Read the model definition and answer for the solid it produces. Units are mm, in the model's axes. A direction names the side the tool comes from. Give positions to 0.01 mm unless a question says otherwise; leave off trailing zeros. Write each loop counter-clockwise with the first axis right and the second up, starting at its lowest first coordinate (ties: lowest second). Pieces come first, ordered by that corner, then holes. Notation, with made-up numbers: (32, 39) - (55, 39) arc R7 cw to (55, 43) - close; hole circle Ø7 at (-35.75, 60). An arc over 180 degrees is marked (long way). Answer as a JSON object with one key per item and string values. Group by question number.
```python
from build123d import *

# Parameters (mm, degrees)
EXTRUDE_THIN1_DEPTH      = 640
EXTRUDE_THIN1_DEPTH_BACK = 640
CUT_EXTRUDE1_DEPTH       = 644.506021728
CUT_EXTRUDE1_DEPTH_BACK  = 644.506021728
SKETCH2_R                = 9


with BuildPart() as part:
    # Sketch1 → Extrude-Thin1 (new, two sides: drawn at the far end of the back side and taken through both)
    with BuildSketch(Plane(origin=(0, 0, 0), x_dir=(0, 0, -1), z_dir=(1, 0, 0)).offset(-EXTRUDE_THIN1_DEPTH_BACK)):
        with BuildLine():
            Line((-30, 50), (-30, -50))
            ThreePointArc((-30, -50), (-27.071067812, -57.071067812), (-20, -60))
            Line((-20, -60), (20, -60))
            ThreePointArc((20, -60), (27.071067812, -57.071067812), (30, -50))
            Line((30, -50), (30, 50))
            ThreePointArc((30, 50), (27.071067812, 57.071067812), (20, 60))
            Line((20, 60), (-20, 60))
            ThreePointArc((-20, 60), (-27.071067812, 57.071067812), (-30, 50))
        make_face()
        with BuildLine():
            Line((-27, 50), (-27, -50))
            ThreePointArc((-27, -50), (-24.949747468, -54.949747468), (-20, -57))
            Line((-20, -57), (20, -57))
            ThreePointArc((20, -57), (24.949747468, -54.949747468), (27, -50))
            Line((27, -50), (27, 50))
            ThreePointArc((27, 50), (24.949747468, 54.949747468), (20, 57))
            Line((20, 57), (-20, 57))
            ThreePointArc((-20, 57), (-24.949747468, 54.949747468), (-27, 50))
        make_face(mode=Mode.SUBTRACT)
    extrude(amount=EXTRUDE_THIN1_DEPTH + EXTRUDE_THIN1_DEPTH_BACK)

    # Sketch2 → Cut-Extrude1 (cut, two sides: drawn at the far end of the back side and taken through both)
    with BuildSketch(Plane.XY.offset(-CUT_EXTRUDE1_DEPTH_BACK)):
        Circle(SKETCH2_R)
        with Locations((-350, 0)):
            Circle(SKETCH2_R)
        with Locations(Location((350, 0, 0), (0, 0, 180))):
            Circle(SKETCH2_R)
    extrude(amount=CUT_EXTRUDE1_DEPTH + CUT_EXTRUDE1_DEPTH_BACK, mode=Mode.SUBTRACT)


solid = part.part
```
1) Find the intervals of material crossed by line 1 (Y direction, x = -120.5, z = 6); line 2 (Z direction, x = -98.5, y = -15); line 3 (Y direction, x = -41, z = 23), in increasing order. Write a range as [from, to].
2) Find section B-B, the plane z = 10.5. Write down the section's boundary in (x, y), and give its area (3 significant figures).
3) A flat-ended cylindrical pin translates along its axis: pin 1 Ø20.5 at (x, y) = (0, 0) entering from -Z. Find the tip coordinate at first contact, or state that the pin passes through.
4) For a pull along Z with two mould halves and no side action, classify faces 1 (the flat face through (-9, 57, 0)), 2 (the flat face through (-640, 0, 29)), 3 (the flat face through (-9, -12, -30)) as released by +Z, released by -Z, zero draft, split by the parting line, or undercut.
5) Find section C-C, the plane x = 197. Write down the section's boundary in (y, z).
6) Find section A-A, the plane y = -20.5. Write down the section's boundary in (x, z).
7) Which of the six approach directions +Z, -Z, +X, -X, +Y, -Y give full straight-line access (tool end or side, diameter ignored) to faces 4 (the flat face through (-9, 12, 30)), 5 (the flat face through (-9, -12, -27))?
Values follow:
{
 "1": {"line 1": "y = [-60, -57], [57, 60]", "line 2": "z = [-30, -27], [27, 30]", "line 3": "y = [-59.54, -56.32], [56.32, 59.54]"},
 "2": {"outline": "(-640, -60) - (640, -60) - (640, -57) - (-640, -57) - close; (-640, 57) - (640, 57) - (640, 60) - (-640, 60) - close", "area": "7,680 mm2"},
 "3": {"pin 1": "stops at z = -30"},
 "4": {"face 1": "undercut", "face 2": "zero draft", "face 3": "released by -Z"},
 "5": {"outline": "(-60, -20) arc R10 ccw to (-50, -30) - (50, -30) arc R10 ccw to (60, -20) - (60, 20) arc R10 ccw to (50, 30) - (-50, 30) arc R10 ccw to (-60, 20) - close; hole (-57, -20) arc R7 ccw to (-50, -27) - (50, -27) arc R7 ccw to (57, -20) - (57, 20) arc R7 ccw to (50, 27) - (-50, 27) arc R7 ccw to (-57, 20) - close"},
 "6": {"outline": "(-640, -30) - (640, -30) - (640, -27) - (-640, -27) - close; (-640, 27) - (640, 27) - (640, 30) - (-640, 30) - close"},
 "7": {"face 4": "+Z, +X, -X, +Y, -Y", "face 5": "+X, -X"}
}
